Geometry: see drawing. Coordinates: mm, zero at the bounding-box minimum. Round coordinates to 2 decimals unless told otherwise and drop trailing zeros. Order: outer loops, then holes, each group sorted by start corner. A loop starts at its lowest first (then second) coordinate and runs counter-clockwise, first axis right, second up. Notation, with made-up numbers: (55.25, 44) -> (103.25, 44) arc R26 ccw to (103.25, 79) -> close; hole circle Ø5 at (64.5, 20). An arc over 180 degrees is marked (long way). Use a Markdown table: item, result.
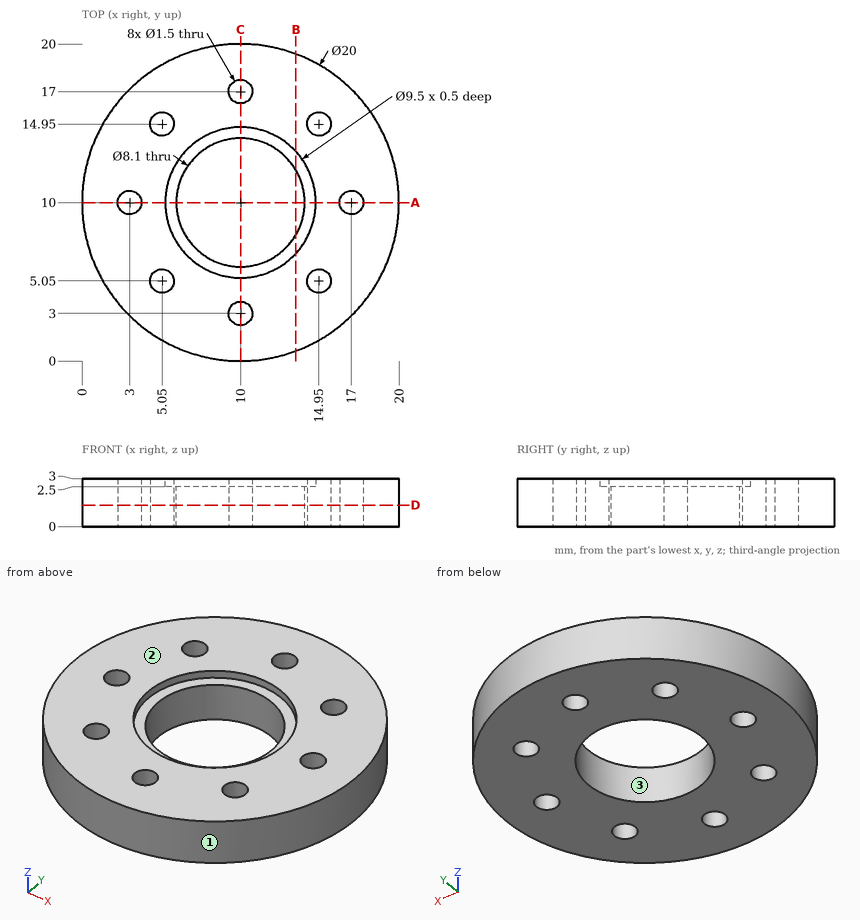
1) Ray query, probe 1 along X at (y, z) = (15.25, 2.8); probe 2 along Y at (x, z) = (9.75, 1.75); probe 3 along Y at (x, z) = (13.25, 0.8) (1 decimal). Return the intervals inside material, ascending.
Answer key:
| item | result |
|---|---|
| probe 1 | x = 1.49 to 4.36, 5.74 to 14.26, 15.64 to 18.51 |
| probe 2 | y = 0 to 2.29, 3.71 to 5.96, 14.04 to 16.29, 17.71 to 20 |
| probe 3 | y = 0.5 to 7.6, 12.4 to 19.5 |
2) Cut plane A-A on y = 10. Return loops of the section in (x, z), and give its area (3 significant figures).
Answer key:
| item | result |
|---|---|
| outline | (0, 0) -> (2.25, 0) -> (2.25, 3) -> (0, 3) -> close; (3.75, 0) -> (5.95, 0) -> (5.95, 2.5) -> (5.25, 2.5) -> (5.25, 3) -> (3.75, 3) -> close; (14.05, 0) -> (16.25, 0) -> (16.25, 3) -> (14.75, 3) -> (14.75, 2.5) -> (14.05, 2.5) -> close; (17.75, 0) -> (20, 0) -> (20, 3) -> (17.75, 3) -> close |
| area | 26.0 mm^2 |
3) Cut plane B-B on x = 13.5. Return loops of the section in (y, z), and give its area (3 significant figures).
Answer key:
| item | result |
|---|---|
| outline | (0.63, 0) -> (7.96, 0) -> (7.96, 2.5) -> (6.79, 2.5) -> (6.79, 3) -> (0.63, 3) -> close; (12.04, 0) -> (19.37, 0) -> (19.37, 3) -> (13.21, 3) -> (13.21, 2.5) -> (12.04, 2.5) -> close |
| area | 42.8 mm^2 |
4) Cut plane D-D on z = 1.35. State how many separate pieces and enclosed holes the cut face has.
Answer key:
| item | result |
|---|---|
| separate pieces | 1 |
| enclosed holes | 9 |
5) Draft query along X for the marked faces 1, 2 and 3. Return one class per face: released by +X, released by -X, zero draft, split by the parting line, or undercut.
Answer key:
| item | result |
|---|---|
| face 1 | split by the parting line |
| face 2 | zero draft |
| face 3 | undercut |
6) Contact query for a flat-ended pin moving along its axis: P1, Ø2, axis at x = 10, y = 3, coming from the +Z side. Output: stop coordinate, or through.
Answer key:
| item | result |
|---|---|
| P1 | stops at z = 3 |
